Input: part model. Units: mm. Frame: model coordinates. Give positions to 0.01 mm unless a question says otherwise; leave off trailing zeros. Loops run counter-clockwise (first coordinate to the right, second up) from the corner with the lowest first, then second, coordinate; pieces in that order, holes last.
from build123d import *

# Parameters (mm, degrees)
SKETCH1_W               = 82.55
SKETCH1_H               = 25.4
BOSS_EXTRUDE1_DEPTH     = 9.525
F_1_4_CLEARANCE_HOLE1_D = 6.5278
SKETCH15_R              = 1.5
CUT_EXTRUDE1_DEPTH      = 26.4


with BuildPart() as part:
    # Sketch1 → Boss-Extrude1 (new body)
    with BuildSketch(Plane(origin=(0, 0, 0), x_dir=(1, 0, 0), z_dir=(0, 1, 0))):
        with Locations((-41.275, -12.7)):
            Rectangle(SKETCH1_W, SKETCH1_H)
    extrude(amount=BOSS_EXTRUDE1_DEPTH)

    # 1/4 Clearance Hole1 (through all)
    with Locations(Plane(origin=(0, 9.525, 0), x_dir=(1, 0, 0), z_dir=(0, 1, 0))):
        with Locations((-73.66, -14.200000048), (-35.56, -14.200000048)):
            Hole(F_1_4_CLEARANCE_HOLE1_D / 2)

    # Sketch15 → Cut-Extrude1 (cut, through all)
    with BuildSketch(Plane.XY.offset(25.4)):
        with Locations((-65.278, 4.7625)):
            Circle(SKETCH15_R)
        with Locations((-10.16, 4.7625)):
            Circle(SKETCH15_R)
    extrude(amount=-CUT_EXTRUDE1_DEPTH, mode=Mode.SUBTRACT)


solid = part.part
(1) Cut plane D-D (x = -10.16). Return the cut outline in (y, z) (1 decimal), and give its area (3 significant figures).
Values follow:
outline: (0, 0) - (3.3, 0) - (3.3, 25.4) - (0, 25.4) - close; (6.3, 0) - (9.5, 0) - (9.5, 25.4) - (6.3, 25.4) - close
area: 166 mm2
(2) Cut plane A-A (y = 4). Return the cut outline in (x, z).
Values follow:
outline: (-82.55, 0) - (-66.57, 0) - (-66.57, 25.4) - (-82.55, 25.4) - close; (-63.99, 0) - (-11.45, 0) - (-11.45, 25.4) - (-63.99, 25.4) - close; (-8.87, 0) - (0, 0) - (0, 25.4) - (-8.87, 25.4) - close; hole circle Ø6.53 at (-73.66, 14.2); hole circle Ø6.53 at (-35.56, 14.2)
(3) Cut plane C-C (x = -35.56). Return the cut outline in (y, z) (3 decimals), and give its area (3 significant figures).
Values follow:
outline: (0, 0) - (9.525, 0) - (9.525, 10.936) - (0, 10.936) - close; (0, 17.464) - (9.525, 17.464) - (9.525, 25.4) - (0, 25.4) - close
area: 180 mm2
(4) Pin query (flat end, axial travel): pin 1 Ø5 at (x, y) = (-46.5, 6) entering from -Z; pin 2 Ø6 at (x, z) = (-35.56, 14.2) entering from -Y. Return the tip coordinate at first contact, or that it passes through.
Values follow:
pin 1: stops at z = 0
pin 2: passes through
(5) Cut plane B-B (z = 14.2). Count the separate pieces of the cut face and the enclosed holes in it, and give its area (3 significant figures).
Values follow:
separate pieces: 3
enclosed holes: 2
area: 648 mm2
(6) Mould query, pull axis Y, two halves, no side actions, for faces 1 (the flat face through (-42, 9.525, 13)), 2 (the flat face through (-42, 5, 0)), 3 (the cylindrical face through (-64.59, 3.43, 12.88)), 4 (the cylindrical face through (-8.774, 4.188, 12.878)). Classes: +Y half, -Y half, draft (parallel to the pull), parting line (faces both ways), or undercut.
Values follow:
face 1: +Y half
face 2: draft
face 3: undercut
face 4: undercut
(7) Ray query, probe 1 along Z at (x, y) = (-73.66, 4.5); probe 2 along X at (y, z) = (1.25, 17); probe 3 along X at (y, z) = (5.25, 2.75). Return the intervals inside material, ascending.
Values follow:
probe 1: z = 0 to 10.94, 17.46 to 25.4
probe 2: x = -82.55 to -75.34, -71.98 to -37.24, -33.88 to 0
probe 3: x = -82.55 to -66.7, -63.86 to -11.58, -8.74 to 0
